For this review, use the dimensioned drawing (mm, ordinates from the lowest corner) and the shaded views. Round coordinates to 2 decimals unless told otherwise and drop trailing zeros. Write each loop counter-clockwise with the first axis right and the second up, starting at its lowest first coordinate (ties: lowest second). Pieces come first, ordered by that corner, then holes.
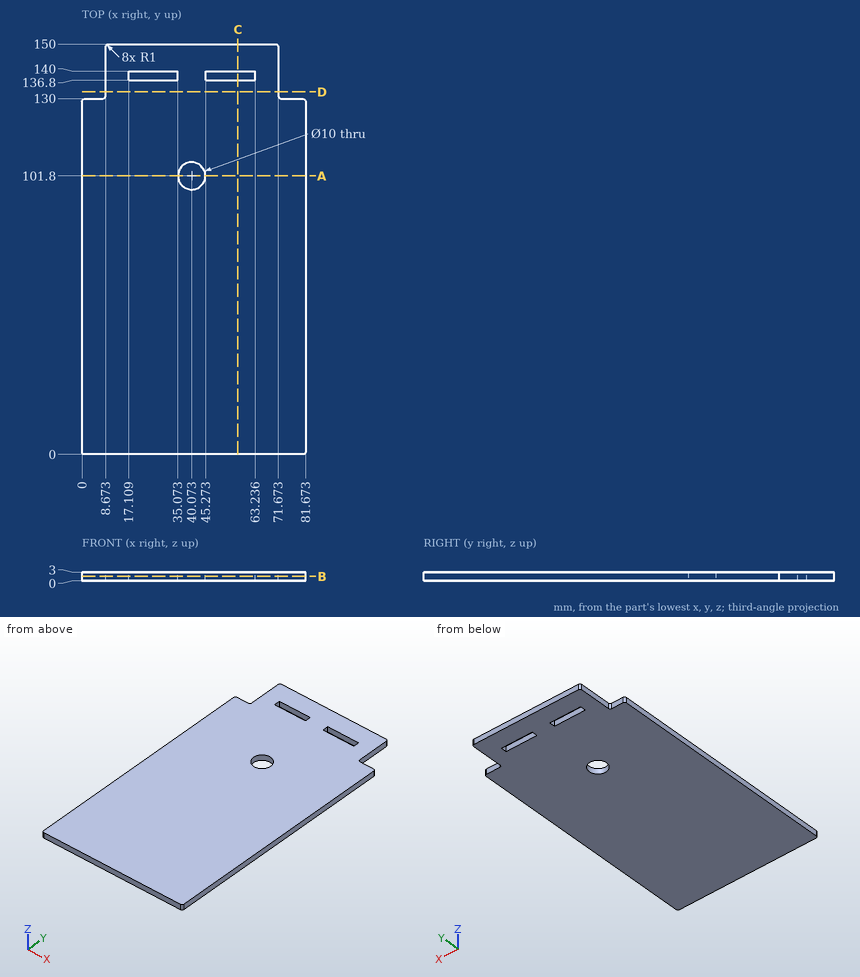
(1) For line 1 along Y through (x, z) = (31.5, 2.2); line 2 along Y through (x, z) = (78, 2.35); line 3 along Y through (x, z) = (39, 2.55), list the stretches that pass through material, from the lowest coordinate up.
Geometry check:
line 1: y = 0 to 136.8, 140 to 150
line 2: y = 0 to 130
line 3: y = 0 to 96.92, 106.68 to 150
(2) We need section B-B, the plane z = 1.55. Give the boundary of the cut face in (x, y), and give its area (3 significant figures).
Geometry check:
outline: (0, 1) arc R1 ccw to (1, 0) - (80.67, 0) arc R1 ccw to (81.67, 1) - (81.67, 129) arc R1 ccw to (80.67, 130) - (72.67, 130) arc R1 cw to (71.67, 131) - (71.67, 149) arc R1 ccw to (70.67, 150) - (9.67, 150) arc R1 ccw to (8.67, 149) - (8.67, 131) arc R1 cw to (7.67, 130) - (1, 130) arc R1 ccw to (0, 129) - close; hole (17.11, 136.8) - (35.07, 136.8) - (35.07, 140) - (17.11, 140) - close; hole circle Ø10 at (40.07, 101.8); hole (45.27, 136.8) - (63.24, 136.8) - (63.24, 140) - (45.27, 140) - close
area: 11,700 mm2
(3) We need section A-A, the plane y = 101.8. Give the boundary of the cut face in (x, z), and give its area (3 significant figures).
Geometry check:
outline: (0, 0) - (35.07, 0) - (35.07, 3) - (0, 3) - close; (45.07, 0) - (81.67, 0) - (81.67, 3) - (45.07, 3) - close
area: 215 mm2
(4) We need section D-D, the plane y = 132.5. Give the boundary of the cut face in (x, z).
Geometry check:
outline: (8.67, 0) - (71.67, 0) - (71.67, 3) - (8.67, 3) - close
(5) For pin 1 Ø8 at (x, y) = (40.07, 101.8) entering from -Z; pin 2 Ø0.9 at (y, z) = (143, 2) entering from +X; pin 3 Ø1.5 at (y, z) = (138, 2) entering from -X, all flat-tipped, find the tip position at first contact; note any pin that passes through.
Geometry check:
pin 1: passes through
pin 2: stops at x = 71.67
pin 3: stops at x = 8.67
(6) We need section C-C, the plane x = 57. Give the boundary of the cut face in (y, z).
Geometry check:
outline: (0, 0) - (136.8, 0) - (136.8, 3) - (0, 3) - close; (140, 0) - (150, 0) - (150, 3) - (140, 3) - close
